```python
from build123d import *

# Parameters (mm, degrees)
SKETCH_1_W               = 33.2
SKETCH_1_H               = 33.2
EXTRUDE_1_DEPTH          = 18
SKETCH_2_W               = 33.2
SKETCH_2_H               = 33.2
EXTRUDE_2_DEPTH          = 2
CUT_EXTRUDE_1_DEPTH      = 40.09219871
CUT_EXTRUDE_1_DEPTH_BACK = 40.09219871
SKETCH_3_W               = 3
SKETCH_3_H               = 6
SKETCH_4_W               = 6
SKETCH_4_H               = 3
CUT_EXTRUDE_2_DEPTH      = 43.163965658
SKETCH_5_W               = 4
SKETCH_5_H               = 6
SKETCH_5_W_2             = 6
SKETCH_5_H_2             = 4
CUT_EXTRUDE_3_DEPTH      = 30.582427216
SKETCH_6_R               = 1.6
CUT_EXTRUDE_4_DEPTH      = 43.163965658
SKETCH_7_R               = 1.55
CUT_EXTRUDE_5_DEPTH      = 43.163965658


with BuildPart() as part:
    # 草图1 → 凸台-拉伸1 (new body)
    with BuildSketch(Plane.XY):
        Rectangle(SKETCH_1_W, SKETCH_1_H)
        with BuildLine():
            Line((11.6, -12.6), (-11.6, -12.6))
            ThreePointArc((-11.6, -12.6), (-12.1, -13.1), (-12.6, -12.6))
            Line((-12.6, -12.6), (-12.6, 12.6))
            ThreePointArc((-12.6, 12.6), (-12.1, 13.1), (-11.6, 12.6))
            Line((-11.6, 12.6), (11.6, 12.6))
            ThreePointArc((11.6, 12.6), (12.1, 13.1), (12.6, 12.6))
            Line((12.6, 12.6), (12.6, -12.6))
            ThreePointArc((12.6, -12.6), (12.1, -13.1), (11.6, -12.6))
        make_face(mode=Mode.SUBTRACT)
    extrude(amount=EXTRUDE_1_DEPTH)

    # 草图2 → 凸台-拉伸2 (add)
    with BuildSketch(Plane.XY.offset(18)):
        Rectangle(SKETCH_2_W, SKETCH_2_H)
    extrude(amount=EXTRUDE_2_DEPTH)

    # 草图3 → 切除-拉伸1 (cut, two sides: drawn at the far end of the back side and taken through both)
    with BuildSketch(Plane(origin=(-12.6, 0, 0), x_dir=(0, 0, -1), z_dir=(1, 0, 0)).offset(-CUT_EXTRUDE_1_DEPTH_BACK)):
        with Locations((-16.5, 0)):
            Rectangle(SKETCH_3_W, SKETCH_3_H)
    extrude(amount=CUT_EXTRUDE_1_DEPTH + CUT_EXTRUDE_1_DEPTH_BACK, mode=Mode.SUBTRACT)

    # 草图4 → 切除-拉伸2 (cut, through all)
    with BuildSketch(Plane(origin=(0, 16.6, 0), x_dir=(1, 0, 0), z_dir=(0, 1, 0))):
        with Locations((0, -16.5)):
            Rectangle(SKETCH_4_W, SKETCH_4_H)
    extrude(amount=-CUT_EXTRUDE_2_DEPTH, mode=Mode.SUBTRACT)

    # 草图5 → 切除-拉伸3 (cut, through all)
    with BuildSketch(Plane(origin=(0, 0, 18), x_dir=(-1, 0, 0), z_dir=(0, 0, -1))):
        with Locations((-14.6, 0)):
            Rectangle(SKETCH_5_W, SKETCH_5_H)
        with Locations((0, -14.6)):
            Rectangle(SKETCH_5_W_2, SKETCH_5_H_2)
        with Locations((14.6, 0)):
            Rectangle(SKETCH_5_W, SKETCH_5_H)
        with Locations((0, 14.6)):
            Rectangle(SKETCH_5_W_2, SKETCH_5_H_2)
    extrude(amount=-CUT_EXTRUDE_3_DEPTH, mode=Mode.SUBTRACT)

    # 草图6 → 切除-拉伸4 (cut, through all)
    with BuildSketch(Plane(origin=(0, 16.6, 0), x_dir=(1, 0, 0), z_dir=(0, 1, 0))):
        with Locations(Location((7.5, -6.9, 0), (0, 0, 270))):
            Circle(SKETCH_6_R)
        with Locations(Location((7.5, -14.9, 0), (0, 0, 270))):
            Circle(SKETCH_6_R)
        with Locations(Location((-7.5, -14.9, 0), (0, 0, 270))):
            Circle(SKETCH_6_R)
        with Locations(Location((-7.5, -6.9, 0), (0, 0, 270))):
            Circle(SKETCH_6_R)
        with Locations(Location((0, -10.9, 0), (0, 0, 270))):
            Circle(SKETCH_6_R)
    extrude(amount=-CUT_EXTRUDE_4_DEPTH, mode=Mode.SUBTRACT)

    # 草图7 → 切除-拉伸5 (cut, through all)
    with BuildSketch(Plane(origin=(16.6, 0, 0), x_dir=(0, 0, -1), z_dir=(1, 0, 0))):
        with Locations((-3.9, -7)):
            Circle(SKETCH_7_R)
        with Locations((-11.9, -7)):
            Circle(SKETCH_7_R)
        with Locations((-11.9, 7)):
            Circle(SKETCH_7_R)
        with Locations((-3.9, 7)):
            Circle(SKETCH_7_R)
    extrude(amount=-CUT_EXTRUDE_5_DEPTH, mode=Mode.SUBTRACT)


solid = part.part
```
Source: CAD feature listing. Evaluate the final solid. Frame: model axes, mm. A direction names the side the tool comes from. Give positions to 0.01 mm unless a question says otherwise; leave off trailing zeros. Loops run counter-clockwise (first coordinate to the right, second up) from the corner with the lowest first, then second, coordinate; pieces in that order, holes last. Notation, with made-up numbers: M -27.5,82.5 L -16.5,82.5 A34 ccw -16.5,118.5 Z; hole C -36,59 d11. An arc over 180 degrees is marked long. Put each result on its own line as item: value.
Q1. Mould query, pull axis Z, two halves, no side actions, for faces 4 (the flat face through (0, 12.6, 9)), 5 (the cylindrical face through (-14.572, 5.625, 11.185)), 6 (the flat face through (-15, 0, 15)). Classes: released by +Z, released by -Z, zero draft, split by the parting line, or undercut.
Response values:
face 4: zero draft
face 5: undercut
face 6: released by +Z
Q2. Reachability of faces 1 (the flat face through (-3, -15, 18)), 2 (the flat face through (0, -15, 15)), 3 (the cylindrical face through (5.94, 14.63, 6.55)) from +Z, -Z, +X, -X, +Y, -Y: full face, straight path, thin tool, end or side. Return the list, or none.
Response values:
face 1: +Z, -Y
face 2: +Z, +Y, -Y
face 3: +Y, -Y
Q3. Section A-A (y = 0). Return the cut outline in (x, z), and give its area (3 significant figures).
Response values:
outline: M -16.6,0 L -12.6,0 L -12.6,15 L -16.6,15 Z; M -12.6,18 L 12.6,18 L 12.6,20 L -12.6,20 Z; M 12.6,0 L 16.6,0 L 16.6,15 L 12.6,15 Z
area: 170 mm²
Q4. Line query: probe 1 along Y at (x, z) = (-15.55, 3.9); probe 2 along X at (y, z) = (13.9, 14.9); probe 3 along Y at (x, z) = (5.5, 15.5). Output: solid intervals per line, ascending. Write a range as [from, to].
Response values:
probe 1: y = [-16.6, -8.55], [-5.45, 5.45], [8.55, 16.6]
probe 2: x = [-16.6, -9.1], [-5.9, 5.9], [9.1, 16.6]
probe 3: y = [-16.6, -12.6], [12.6, 16.6]
Q5. Pin query (flat end, axial travel): P1, Ø5, axis at y = 7, z = 11.9, coming from the -X side; P2, Ø2.5, axis at x = 7.5, z = 6.9, coming from the +Y side (3 decimals); P3, Ø12.5, axis at x = -6, y = -3, coming from the -Z side; P4, Ø2, axis at x = -1.5, z = 19.5, coming from the -Y side. Return the tip coordinate at first contact, or that it passes through.
Response values:
P1: stops at x = -16.6
P2: passes through
P3: stops at z = 18
P4: stops at y = -12.6
Q6. Section C-C (x = 0). Return the cut outline in (y, z).
Response values:
outline: M -16.6,0 L -12.6,0 L -12.6,9.3 L -16.6,9.3 Z; M -16.6,12.5 L -12.6,12.5 L -12.6,15 L -16.6,15 Z; M -12.6,18 L 12.6,18 L 12.6,20 L -12.6,20 Z; M 12.6,0 L 16.6,0 L 16.6,9.3 L 12.6,9.3 Z; M 12.6,12.5 L 16.6,12.5 L 16.6,15 L 12.6,15 Z
Q7. Section B-B (z = 1.75). Return the cut outline in (x, y).
Response values:
outline: M -16.6,-16.6 L 16.6,-16.6 L 16.6,16.6 L -16.6,16.6 Z; hole M -12.6,-12.6 A0.5 ccw -11.6,-12.6 L 11.6,-12.6 A0.5 ccw 12.6,-12.6 L 12.6,12.6 A0.5 ccw 11.6,12.6 L -11.6,12.6 A0.5 ccw -12.6,12.6 Z
Q8. Section D-D (y = -7). Return the cut outline in (x, z).
Response values:
outline: M -16.6,0 L -12.6,0 L -12.6,2.35 L -16.6,2.35 Z; M -16.6,5.45 L -12.6,5.45 L -12.6,10.35 L -16.6,10.35 Z; M -16.6,13.45 L -12.6,13.45 L -12.6,18 L 12.6,18 L 12.6,13.45 L 16.6,13.45 L 16.6,20 L -16.6,20 Z; M 12.6,0 L 16.6,0 L 16.6,2.35 L 12.6,2.35 Z; M 12.6,5.45 L 16.6,5.45 L 16.6,10.35 L 12.6,10.35 Z
